Can you work these out from the model? Positions are in its coordinate system, mm. A direction names the side the tool comes from. Round coordinates to 2 decimals unless told otherwise and drop trailing zeros. Loops run counter-clockwise (first coordinate to the right, second up) from the corner with the lowest first, then second, coordinate; pieces in that order, holes last. Notation, with made-up numbers: (-15.75, 78) - (24.25, 78) arc R37 ccw to (24.25, 115) - close; hole circle Ø7 at (-19.5, -6). An arc over 180 degrees is marked (long way). Answer as CSV lines item,"result".
```python
from build123d import *

# Parameters (mm, degrees)
F1_DEPTH    = 20
F2_W        = 18
F2_H        = 1.6
F3_DEPTH    = 8.1
F4_R        = 1.2
F5_T1_DEPTH = 29.1153030611
F5_T3_DEPTH = 31.6404483572
F5_T5_DEPTH = 45


# Not quite as in the source:
# - a fillet or chamfer that OpenCascade refuses, or shapes differently, is made with other operations: its cross-section is extruded or revolved along the edge and cut away or added


with BuildPart() as f1:
    # F0 (on Top) → F1 (new body)
    with BuildSketch(Plane.XY):
        Polygon((-24, 0.2), (-8.5, 0.2), (0, 0.2), (0, 1.7), (0, 13.8), (-8.5, 13.8), (-8.5, 15), (-100, 15), (-100, 8), (-96.9, 5.3927982226), (-94.9, 5.3927982226), (-94.9, 8.3), (-24, 8.3), align=None)
    extrude(amount=F1_DEPTH)

    # F2 (on face) → F3 (join)
    with BuildSketch(Plane.XZ.offset(-8.3)):
        with Locations((-33, 19.2)):
            Rectangle(F2_W, F2_H)
    extrude(amount=F3_DEPTH)

    # F4
    f4_edges = [f1.edges().sort_by_distance(p)[0] for p in [
        (-42, 4.25, 18.4),
    ]]
    fillet(f4_edges, radius=F4_R)

    # F5: fillet of radius 5 on 3 edges, made by hand

    # F5_s2 → F5_t1 (cut)
    with BuildSketch(Plane.XY.offset(-4.5576515305)):
        with BuildLine():
            ThreePointArc((-98.2952164267, 6.5662210444), (-96.7897023762, 5.6953049607), (-95.0769393878, 5.3927982226))
            Line((-95.0769393878, 5.3927982226), (-96.9, 5.3927982226))
            Line((-96.9, 5.3927982226), (-98.2952164267, 6.5662210444))
        make_face()
    extrude(amount=F5_T1_DEPTH, mode=Mode.SUBTRACT)

    # F5_s4 → F5_t3 (cut)
    with BuildSketch(Plane.XY.offset(-5.8202241786)):
        with BuildLine():
            ThreePointArc((-100, 10.3280896714), (-99.5327356637, 8.217566655), (-98.2182770389, 6.5015124932))
            Line((-98.2182770389, 6.5015124932), (-100, 8))
            Line((-100, 8), (-100, 10.3280896714))
        make_face()
    extrude(amount=F5_T3_DEPTH, mode=Mode.SUBTRACT)

    # F5_s6 → F5_t5 (cut)
    with BuildSketch(Plane.XY.offset(-12.5)):
        with BuildLine():
            ThreePointArc((-95, 15), (-98.5355339059, 13.5355339059), (-100, 10))
            Line((-100, 10), (-100, 15))
            Line((-100, 15), (-95, 15))
        make_face()
    extrude(amount=F5_T5_DEPTH, mode=Mode.SUBTRACT)


solid = f1.part
```
Q1. We'd pull the mould along X, two halves only. Please class faces 4 (the flat face through (-4, 13.8, 10)), 5 (the flat face through (-60, 8.3, 10)), 6 (the flat face through (0, 7, 10)): pulls with the +X half, pulls with the -X half, needs draft (parallel to the pull), parting line crosses it, or undercut.
Checks:
face 4,"needs draft"
face 5,"undercut"
face 6,"pulls with the +X half"
Q2. I'm going to push flat-ended pins straight in: pin 1 Ø2.5 at (x, y) = (-30, 4.5) entering from -Z; pin 2 Ø3 at (y, z) = (5.5, 13.5) entering from -X. Where does each tip first touch, or does it pass through?
Checks:
pin 1,"z = 18.4"
pin 2,"x = -98.73"
Q3. On a 3-axis mill with a long thin cutter (end or side, diameter ignored), from which of +Z, -Z, +X, -X, +Y, -Y can I reach the whole of each face in a straight line? I mean faces 1 (the flat face through (-33, 4, 18.4)), 2 (the flat face through (-40, 9, 20)), 3 (the flat face through (-94.9, 7, 10)). Say none if no direction works.
Checks:
face 1,"-Z, -Y"
face 2,"+Z, +X, -X, +Y, -Y"
face 3,"+Z, -Z, -Y"
Q4. If I drill on line 1 along Y through (x, z) = (-27.5, 17.5); line 2 along X through (y, z) = (7.25, 1); line 3 along X through (y, z) = (3.75, 2.5), over which ranges is the centre line in solid material (lowest first)? Write a range as [from, to].
Checks:
line 1,"[8.3, 15]"
line 2,"[-98.94, -94.9], [-24, 0]"
line 3,"[-24, 0]"
Q5. Imagine slicing it at C-C (x = -25). Write out the boundary of the cut face in (y, z).
Checks:
outline,"(0.2, 18.4) - (8.3, 18.4) - (8.3, 0) - (15, 0) - (15, 20) - (0.2, 20) - close"
Q6. Imagine slicing it at A-A (y = 3). Write out the boundary of the cut face in (x, z), then the cut area to 3 significant figures.
Checks:
outline,"(-42, 19.6) arc R1.2 ccw to (-40.8, 18.4) - (-24, 18.4) - (-24, 0) - (0, 0) - (0, 20) - (-42, 20) - close"
area,"508 mm²"
Q7. Imagine slicing it at D-D (x = -53.5). Write out the boundary of the cut face in (y, z).
Checks:
outline,"(8.3, 0) - (15, 0) - (15, 20) - (8.3, 20) - close"
Q8. Imagine slicing it at B-B (z = 2). Write out the boundary of the cut face in (x, y).
Checks:
outline,"(-100, 10.16) arc R5 ccw to (-98.26, 6.53) arc R5 ccw to (-95.08, 5.39) - (-94.9, 5.39) - (-94.9, 8.3) - (-24, 8.3) - (-24, 0.2) - (0, 0.2) - (0, 13.8) - (-8.5, 13.8) - (-8.5, 15) - (-95, 15) arc R5 ccw to start"
